from build123d import *

# Parameters (mm, degrees)
F0_R     = 40
F1_DEPTH = 25
F2_DEPTH = 10
F4_DEPTH = 5


with BuildPart() as f1:
    # F0 (on Right) → F1 (new body, symmetric)
    with BuildSketch(Plane.YZ):
        with BuildLine():
            ThreePointArc((-15, 42.426407), (-25.980762, -36.742346), (45, 0))
            ThreePointArc((45, 0), (36.742346, 25.980762), (15, 42.426407))
            ThreePointArc((15, 42.426407), (0, 45), (-15, 42.426407))
        make_face()
        Circle(F0_R, mode=Mode.SUBTRACT)
    extrude(amount=F1_DEPTH, both=True)

    # F0 (on Right) → F2 (join, symmetric)
    with BuildSketch(Plane.YZ):
        with BuildLine():
            ThreePointArc((-15, 42.426407), (0, 45), (15, 42.426407))
            Line((15, 42.426407), (15, 55))
            Line((15, 55), (-15, 55))
            Line((-15, 55), (-15, 42.426407))
        make_face()
    extrude(amount=F2_DEPTH, both=True)

    # F3 (on Front) → F4 (join, symmetric)
    with BuildSketch(Plane.XZ):
        with BuildLine():
            ThreePointArc((-5, 60.635083), (0, 60), (5, 60.635083))
            ThreePointArc((5, 60.635083), (15.811388, 67.752551), (20, 80))
            ThreePointArc((20, 80), (-12.247449, 95.811388), (-5, 60.635083))
        make_face()
        with BuildLine():
            Line((-5, 55), (5, 55))
            Line((5, 55), (5, 60.635083))
            ThreePointArc((5, 60.635083), (0, 60), (-5, 60.635083))
            Line((-5, 60.635083), (-5, 55))
        make_face()
    extrude(amount=F4_DEPTH, both=True)


solid = f1.part
Here's how the part is built. I have some questions about the finished solid (model axes, mm). A direction names the side the tool comes from. Give positions to 0.01 mm unless a question says otherwise; leave off trailing zeros. Write each loop counter-clockwise with the first axis right and the second up, starting at its lowest first coordinate (ties: lowest second). Pieces come first, ordered by that corner, then holes. Notation, with made-up numbers: (-2.5, 85.25) -> (40.5, 85.25) arc R20 ccw to (40.5, 107.25) -> close; hole circle Ø6 at (60.25, 14.5). An arc over 180 degrees is marked (long way). Use one line per item in the form item = value. Start each with the question number.
1. Imagine slicing it at B-B on y = 0. List the corners of the cut face in (x, z) for me, plus the area to 3 significant figures.
2. Imagine slicing it at D-D on y = 27. List the corners of the cut face in (x, z) for me.
3. Thinking about a two-plate mould opening in Z: for faces 4 (the face through (-5, 0, 58)), 5 (the face through (25, -30.2, -26.5)), which applies, +Z half, -Z half, draft (parallel to the pull), parting line (faces both ways), or undercut?
4. On a 3-axis mill with a long thin cutter (end or side, diameter ignored), from which of +Z, -Z, +X, -X, +Y, -Y can I reach the whole of each face in a straight line? I mean faces 1 (the face through (0, -15, 49)), 2 (the face through (0, 5, 78)), 3 (the face through (5, 0, 58)). Say none if no direction works.
5. Will these pins go through, and if not, where does the flat tip stop? pin 1 Ø4 at (y, z) = (7, 47.5) entering from +X; pin 2 Ø8 at (x, z) = (19, 18) entering from +Y; pin 3 Ø4 at (x, y) = (0.5, 34.5) entering from +Z; pin 4 Ø1.5 at (x, z) = (11.5, 61) entering from +Y.
6. Imagine slicing it at A-A on x = 0. List the corners of the cut face in (y, z) for me.
7. Imagine slicing it at C-C on z = -26. List the corners of the cut face in (x, y) for me.
8. If I drill on L1, parallel to Z at x = 12.5, y = 0; L2, parallel to Z at x = 4.5, y = -21; L3, parallel to Z at x = 9, y = 0, over which ranges is the centre line in solid material (lowest first)?
Entries:
q1.outline = (-25, -45) -> (25, -45) -> (25, -40) -> (-25, -40) -> close; (-25, 40) -> (25, 40) -> (25, 45) -> (10, 45) -> (10, 55) -> (5, 55) -> (5, 60.64) arc R20 ccw (long way) to (-5, 60.64) -> (-5, 55) -> (-10, 55) -> (-10, 45) -> (-25, 45) -> close
q1.area = 2,010 mm²
q2.outline = (-25, -36) -> (25, -36) -> (25, -29.51) -> (-25, -29.51) -> close; (-25, 29.51) -> (25, 29.51) -> (25, 36) -> (-25, 36) -> close
q3.face_4 = undercut
q3.face_5 = draft
q4.face_1 = +Z, +X, -X, -Y
q4.face_2 = +Z, +X, -X, +Y
q4.face_3 = +X, +Y, -Y
q5.pin_1 = 10
q5.pin_2 = 42.77
q5.pin_3 = 31.12
q5.pin_4 = through
q6.outline = (-15, 42.43) arc R45 ccw (long way) to (45, 0) arc R45 ccw to (15, 42.43) -> (15, 55) -> (5, 55) -> (5, 100) -> (-5, 100) -> (-5, 55) -> (-15, 55) -> close; hole circle Ø80 at (0, 0)
q7.outline = (-25, -36.73) -> (25, -36.73) -> (25, -30.4) -> (-25, -30.4) -> close; (-25, 30.4) -> (25, 30.4) -> (25, 36.73) -> (-25, 36.73) -> close
q8.L1 = -45 to -40, 40 to 45, 64.39 to 95.61
q8.L2 = -39.8 to -34.04, 34.04 to 39.8
q8.L3 = -45 to -40, 40 to 55, 62.14 to 97.86
